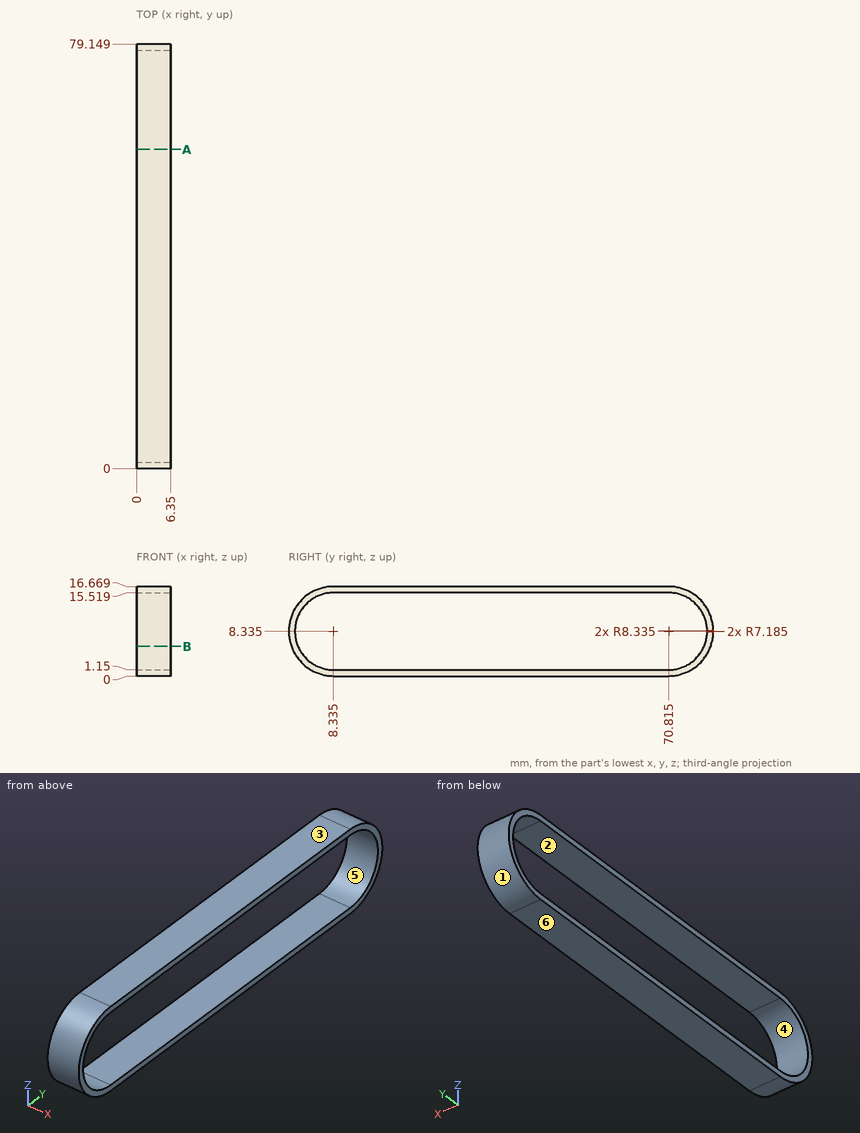
Geometry check sheet. Reference: drawing and pictorial views, mm from the part's lowest x, y, z. A direction names the side the tool comes from. Round coordinates to 2 decimals unless told otherwise and drop trailing zeros. Loops run counter-clockwise (first coordinate to the right, second up) from the corner with the lowest first, then second, coordinate; pieces in that order, holes last. Notation, with made-up numbers: (41, -34.5) -> (100, -34.5) arc R26 ccw to (100, -15.5) -> close; hole circle Ø8 at (67.5, -16.5). An arc over 180 degrees is marked (long way). Answer as a JSON object with one key per item and string values. Group by question number.
Item 1: Set-up check for the marked faces 5 and 6: record each of +Z, -Z, +X, -X, +Y, -Y from which the full face is reachable in a straight line by a thin tool's end or side.
Item 2: Cross-section at A-A, the plane y = 59.5. Record the cut outline in (x, z).
Item 3: Cross-section at B-B, the plane z = 5.5. Record the cut outline in (x, y).
Item 4: Depth check by flat-ended pin: pin 1 Ø10 at (y, z) = (16.5, 3.5) entering from -X. Enter the tip coordinate at first touch or a pass-through.
Item 5: Thickness scan on line 1 along Z through (x, y) = (3.5, 68); line 2 along Y through (x, z) = (5.5, 8.25); line 3 along Y through (x, z) = (4.75, 4) (1 decimal). Record the ranges inside material, lowest first.
Item 6: Release check for a two-part mould opening along Y. For the marked faces 1, 2, 3 and 4 record: pulls with the +Y half, pulls with the -Y half, needs draft (parallel to the pull), parting line crosses it, or undercut.
Determined:
{
 "1": {"face 5": "+X, -X", "face 6": "-Z, +X, -X, +Y, -Y"},
 "2": {"outline": "(0, 0) -> (6.35, 0) -> (6.35, 1.15) -> (0, 1.15) -> close; (0, 15.52) -> (6.35, 15.52) -> (6.35, 16.67) -> (0, 16.67) -> close"},
 "3": {"outline": "(0, 0.5) -> (6.35, 0.5) -> (6.35, 1.73) -> (0, 1.73) -> close; (0, 77.42) -> (6.35, 77.42) -> (6.35, 78.65) -> (0, 78.65) -> close"},
 "4": {"pin 1": "stops at x = 0"},
 "5": {"line 1": "z = 0 to 1.15, 15.52 to 16.67", "line 2": "y = 0 to 1.15, 78 to 79.15", "line 3": "y = 1.2 to 2.6, 76.5 to 77.9"},
 "6": {"face 1": "pulls with the +Y half", "face 2": "undercut", "face 3": "needs draft", "face 4": "undercut"}
}
